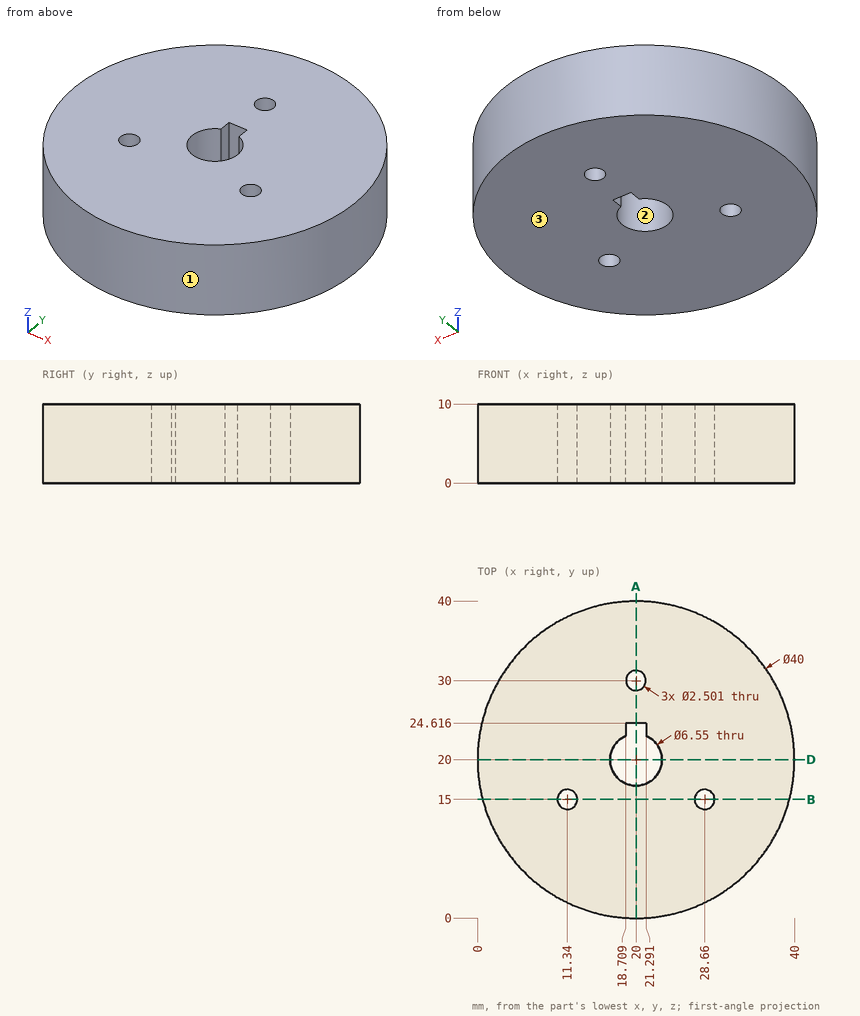
Drawing for the job (mm, zero at the part's lowest x, y, z). Coordinates: 2 decimals unless noted, no trailing zeros. Order: outer loops, then holes, each group sorted by start corner. A loop starts at its lowest first (then second) coordinate and runs counter-clockwise, first axis right, second up. Notation, with made-up numbers: (12, 88.25) -> (69, 88.25) arc R27 ccw to (69, 127.25) -> close; hole circle Ø7 at (53.5, 13.5). An arc over 180 degrees is marked (long way). Return JSON: item names as keys, results as strings.
Item 1: Slice it at B-B (y = 15). Write the cut outline in (x, z) (1 decimal).
Model answer:
{"outline": "(0.6, 0) -> (10.1, 0) -> (10.1, 10) -> (0.6, 10) -> close; (12.6, 0) -> (27.4, 0) -> (27.4, 10) -> (12.6, 10) -> close; (29.9, 0) -> (39.4, 0) -> (39.4, 10) -> (29.9, 10) -> close"}
Item 2: Pin check, flat tips, straight feed: P1, Ø3, axis at x = 13, z = 2.5, coming from the +Y side; P2, Ø0.5, axis at y = 23.5, z = 3, coming from the +X side; P3, Ø1.5, axis at y = 25, z = 8.5, coming from the +X side. Stop position of each tip, or through.
Model answer:
{"P1": "stops at y = 39.23", "P2": "stops at x = 39.73", "P3": "stops at x = 39.54"}
Item 3: Mould opens along X. For the marked faces 1, 2 and 3 say: pulls with the +X half, pulls with the -X half, needs draft (parallel to the pull), parting line crosses it, or undercut.
Model answer:
{"face 1": "parting line crosses it", "face 2": "undercut", "face 3": "needs draft"}
Item 4: Wall check: line 1 along Y through (x, z) = (19.5, 3.5) (1 decimal); line 2 along X through (y, z) = (17, 3.75) (1 decimal); line 3 along Y through (x, z) = (10, 0.75). Give the ranges that are in metal, low to high. Write a range as from..to.
Model answer:
{"line 1": "y = 0..16.8, 24.6..28.9, 31.1..40", "line 2": "x = 0.2..18.7, 21.3..39.8", "line 3": "y = 2.68..37.32"}
Item 5: Slice it at A-A (x = 20). Count the separate pieces of the cut face and the enclosed holes in it, then the cut area to 3 significant figures.
Model answer:
{"separate pieces": "3", "enclosed holes": "0", "area": "296 mm²"}
Item 6: Slice it at D-D (y = 20). Write the cut outline in (x, z) (1 decimal).
Model answer:
{"outline": "(0, 0) -> (16.7, 0) -> (16.7, 10) -> (0, 10) -> close; (23.3, 0) -> (40, 0) -> (40, 10) -> (23.3, 10) -> close"}
